For this review, take the finished solid that the model builds, in its own axes (mm). A direction names the side the tool comes from. Give positions to 0.01 mm unless a question says otherwise; leave off trailing zeros. Write each loop counter-clockwise with the first axis right and the second up, starting at its lowest first coordinate (ties: lowest second). Pieces come first, ordered by that corner, then holes. Notation, with made-up numbers: (-21.75, 88) -> (8.25, 88) arc R16 ccw to (8.25, 109) -> close; hole circle Ø1 at (-9.75, 46). An arc over 180 degrees is marked (long way). Answer as CSV lines item,"result".
```python
from build123d import *

# Parameters (mm, degrees)
SKETCH1_W           = 128
SKETCH1_H           = 40
BOSS_EXTRUDE1_DEPTH = 8
SKETCH2_W           = 128
SKETCH2_H           = 40
BOSS_EXTRUDE2_DEPTH = 30
CUT_EXTRUDE1_DEPTH  = 200000
SKETCH5_W           = 4
SKETCH5_H           = 40
CUT_EXTRUDE2_DEPTH  = 14
SKETCH6_W           = 40
SKETCH6_H           = 35
BOSS_EXTRUDE3_DEPTH = 4
SKETCH7_R           = 6
CUT_EXTRUDE3_DEPTH  = 4
CUT_EXTRUDE3_DRAFT  = 39
SKETCH8_W           = 5
SKETCH8_H           = 2.2
CUT_EXTRUDE4_DEPTH  = 200
SKETCH9_W           = 132
SKETCH9_H           = 5
BOSS_EXTRUDE4_DEPTH = 3
BOSS_EXTRUDE7_DEPTH = 3
BOSS_EXTRUDE9_DEPTH = 3
SKETCH13_R          = 1.5
CUT_EXTRUDE5_DEPTH  = 10


with BuildPart() as part:
    # Sketch1 → Boss-Extrude1 (new body)
    with BuildSketch(Plane(origin=(0, 0, 0), x_dir=(1, 0, 0), z_dir=(0, 1, 0))):
        Rectangle(SKETCH1_W, SKETCH1_H)
    extrude(amount=BOSS_EXTRUDE1_DEPTH)

    # Sketch2 → Boss-Extrude2 (add)
    with BuildSketch(Plane(origin=(0, 8, 0), x_dir=(1, 0, 0), z_dir=(0, 1, 0))):
        Rectangle(SKETCH2_W, SKETCH2_H)
    extrude(amount=BOSS_EXTRUDE2_DEPTH)

    # Sketch3 → Cut-Extrude1 (cut)
    with BuildSketch(Plane(origin=(64, 0, 0), x_dir=(0, 0, -1), z_dir=(1, 0, 0))):
        with BuildLine():
            Line((-15, 19), (-20, 19))
            Line((-20, 19), (-20, 38))
            Line((-20, 38), (20, 38))
            Line((20, 38), (20, 19))
            Line((20, 19), (15, 19))
            ThreePointArc((15, 19), (0, 4), (-15, 19))
        make_face()
    extrude(amount=-CUT_EXTRUDE1_DEPTH, mode=Mode.SUBTRACT)

    # Sketch5 → Cut-Extrude2 (cut)
    with BuildSketch(Plane(origin=(0, 19, 0), x_dir=(1, 0, 0), z_dir=(0, 1, 0))):
        with Locations((-58, 0)):
            Rectangle(SKETCH5_W, SKETCH5_H)
    extrude(amount=-CUT_EXTRUDE2_DEPTH, mode=Mode.SUBTRACT)

    # Sketch6 → Boss-Extrude3 (add)
    with BuildSketch(Plane(origin=(64, 0, 0), x_dir=(0, 0, -1), z_dir=(1, 0, 0))):
        with Locations((0, 17.5)):
            Rectangle(SKETCH6_W, SKETCH6_H)
    extrude(amount=BOSS_EXTRUDE3_DEPTH)


with BuildPart() as cut_extrude3_tool:
    # Sketch7 → Cut-Extrude3 (with draft: the straight prism first)
    with BuildSketch(Plane(origin=(68, 0, 0), x_dir=(0, 0, -1), z_dir=(1, 0, 0))):
        with Locations((0, 19)):
            Circle(SKETCH7_R)
    extrude(amount=-CUT_EXTRUDE3_DEPTH)
    # Cut-Extrude3: the draft: its side faces are tilted about the plane it starts from
    cut_extrude3_sides = [cut_extrude3_tool.faces().sort_by_distance(p)[0] for p in [
        (66, 19, 6),
    ]]
    draft(cut_extrude3_sides, Plane(origin=(68, 0, 0), x_dir=(0, 0, -1), z_dir=(1, 0, 0)), CUT_EXTRUDE3_DRAFT)


with BuildPart() as part_1:
    add(part.part)

    # Cut-Extrude3: cut by cut_extrude3_tool
    add(cut_extrude3_tool.part, mode=Mode.SUBTRACT)

    # Sketch8 → Cut-Extrude4 (cut)
    with BuildSketch(Plane(origin=(0, 0, -20), x_dir=(-1, 0, 0), z_dir=(0, 0, -1))):
        with Locations((-35.5, 3.1)):
            Rectangle(SKETCH8_W, SKETCH8_H)
        with Locations((34.5, 3.1)):
            Rectangle(SKETCH8_W, SKETCH8_H)
        with Locations((-0.5, 3.1)):
            Rectangle(SKETCH8_W, SKETCH8_H)
    extrude(amount=-CUT_EXTRUDE4_DEPTH, mode=Mode.SUBTRACT)

    # Sketch9 → Boss-Extrude4 (add)
    with BuildSketch(Plane.XZ):
        with Locations((2, 22.5)):
            Rectangle(SKETCH9_W, SKETCH9_H)
        with Locations((2, -22.5)):
            Rectangle(SKETCH9_W, SKETCH9_H)
    extrude(amount=-BOSS_EXTRUDE4_DEPTH)

    # Sketch10 → Boss-Extrude7 (add)
    with BuildSketch(Plane.XY.offset(20)):
        Polygon((68, 35), (64, 35), (52, 19), (68, 19), align=None)
    extrude(amount=-BOSS_EXTRUDE7_DEPTH)

    # Sketch12 → Boss-Extrude9 (add)
    with BuildSketch(Plane(origin=(0, 0, -20), x_dir=(-1, 0, 0), z_dir=(0, 0, -1))):
        Polygon((-68, 35), (-64, 35), (-51.978791145, 19), (-68, 19), align=None)
    extrude(amount=-BOSS_EXTRUDE9_DEPTH)

    # Sketch13 → Cut-Extrude5 (cut)
    with BuildSketch(Plane(origin=(0, 3, 0), x_dir=(1, 0, 0), z_dir=(0, 1, 0))):
        with Locations(Location((-59, -22.5, 0), (0, 0, 270))):
            Circle(SKETCH13_R)
        with Locations(Location((-59, 22.5, 0), (0, 0, 270))):
            Circle(SKETCH13_R)
        with Locations(Location((63, -22.5, 0), (0, 0, 270))):
            Circle(SKETCH13_R)
        with Locations(Location((63, 22.5, 0), (0, 0, 270))):
            Circle(SKETCH13_R)
    extrude(amount=-CUT_EXTRUDE5_DEPTH, mode=Mode.SUBTRACT)


solid = part_1.part
```
Q1. Add section A-A (z = -22.5). Write out the cut boundary in (x, y), plus the area to 3 significant figures.
Answer block:
outline,"(-64, 0) -> (-60.5, 0) -> (-60.5, 3) -> (-64, 3) -> close; (-57.5, 0) -> (61.5, 0) -> (61.5, 3) -> (-57.5, 3) -> close; (64.5, 0) -> (68, 0) -> (68, 3) -> (64.5, 3) -> close"
area,"378 mm2"
Q2. To check wall thickness, follow probe 1 along X at (y, z) = (1.1, 22.5); probe 2 along X at (y, z) = (9, -14.5); probe 3 along X at (y, z) = (25, -11.5). State the ranges of each line that lie inside material, in increasing order. Write a range as [from, to].
Answer block:
probe 1,"x = [-64, -60.5], [-57.5, 61.5], [64.5, 68]"
probe 2,"x = [-64, -60], [-56, 68]"
probe 3,"x = [64, 68]"
Q3. Add section C-C (z = -12.5). Write out the cut boundary in (x, y).
Answer block:
outline,"(-64, 0) -> (68, 0) -> (68, 35) -> (64, 35) -> (64, 10.71) -> (-56, 10.71) -> (-56, 5) -> (-60, 5) -> (-60, 10.71) -> (-64, 10.71) -> close; hole (-37, 2) -> (-32, 2) -> (-32, 4.2) -> (-37, 4.2) -> close; hole (-2, 2) -> (3, 2) -> (3, 4.2) -> (-2, 4.2) -> close; hole (33, 2) -> (38, 2) -> (38, 4.2) -> (33, 4.2) -> close"
Q4. Add section D-D (y = 11). State how many separate pieces and enclosed holes the cut face has, plus the area to 3 significant figures.
Answer block:
separate pieces,"3"
enclosed holes,"0"
area,"1,960 mm2"
Q5. For faces 5 (the flat face through (-56, 11, -16)), 6 (the flat face through (36, 4.2, 11)), 7 (the flat face through (-34, 2, 0)), 8 (the cylindrical face through (0.9, 5.02, -5.44)), list the 3-axis set-ups (+Z, -Z, +X, -X, +Y, -Y) from which the entire face can be reached by the end or side of a thin tool; tool diameter is ignored.
Answer block:
face 5,"+Z, -Z, +Y"
face 6,"+Z, -Z"
face 7,"none"
face 8,"-X, +Y"
Q6. Add section B-B (x = 6). Write out the cut boundary in (y, z).
Answer block:
outline,"(0, -25) -> (3, -25) -> (3, -20) -> (19, -20) -> (19, -15) arc R15 cw to (19, 15) -> (19, 20) -> (3, 20) -> (3, 25) -> (0, 25) -> close"
Q7. Draft analysis for pull direction Y (two halves, no side actions). For faces 1 (the flat face through (1, 1, -25)), 2 (the flat face through (38, 3, 0)), 3 (the flat face through (58.07, 27.11, -18.52)), 4 (the flat face through (-32, 3, 0)), state which applies: released by +Y, released by -Y, zero draft, split by the parting line, or undercut.
Answer block:
face 1,"zero draft"
face 2,"undercut"
face 3,"released by +Y"
face 4,"undercut"
Q8. Clearance check with flat-ended pins moving along their axes: pin 1 (1 mm diameter, centred on x = -12.5, y = 18.5, fed in from +Z); pin 2 (6 mm diameter, centred on x = 3, z = 14.5, fed in from +Y); pin 3 (1.5 mm diameter, centred on x = 36, z = 3.5, fed in from +Y). State where each tip first meets the part, or that it passes through.
Answer block:
pin 1,"stops at z = 20"
pin 2,"stops at y = 19"
pin 3,"stops at y = 4.61"
